CAD build for the part. Positions are in the model's coordinates, mm. A direction names the side the tool comes from. Give positions to 0.01 mm unless a question says otherwise; leave off trailing zeros. Loops run counter-clockwise (first coordinate to the right, second up) from the corner with the lowest first, then second, coordinate; pieces in that order, holes last. Notation, with made-up numbers: M 77.25,29.5 L 112.25,29.5 A19 ccw 112.25,48.5 Z; hole C 81.25,14 d9. An arc over 180 degrees is marked long. Answer as CSV lines item,"result".
```python
from build123d import *

# Parameters (mm, degrees)
SKETCH3_R          = 3
CUT_EXTRUDE1_DEPTH = 5


with BuildPart() as part:
    # Sketch1 → Revolve1 (revolve)
    with BuildSketch(Plane.XY, mode=Mode.PRIVATE) as revolve1_sk:
        Polygon((-15.060768988, 23.176328976), (-19, 22.481736265), (-19, 19.651328976), (-10.35, -0.323671024), (-8.6, -0.323671024), (-8.6, -6.823671024), (-5.6, -6.823671024), (-5.6, 3.426328976), (-3, 3.426328976), (-3, -1.573671024), (0, -1.573671024), (0, 23.176328976), align=None)
    revolve(revolve1_sk.sketch.rotate(Axis((0, -1.573671024, 0), (0, 1, 0)), 270), axis=Axis((0, -1.573671024, 0), (0, 1, 0)))

    # Sketch3 → Cut-Extrude1 (cut)
    with BuildSketch(Plane.XZ.offset(1.573671024)):
        Circle(SKETCH3_R)
    extrude(amount=-CUT_EXTRUDE1_DEPTH, mode=Mode.SUBTRACT)


solid = part.part
```
Q1. Cut at A-A (z = 0). Write the cut outline in (x, y), and give its area (3 significant figures).
Solution:
outline,"M -19,19.65 L -10.35,-0.32 L -8.6,-0.32 L -8.6,-6.82 L -5.6,-6.82 L -5.6,3.43 L 5.6,3.43 L 5.6,-6.82 L 8.6,-6.82 L 8.6,-0.32 L 10.35,-0.32 L 19,19.65 L 19,22.48 L 15.06,23.18 L -15.06,23.18 L -19,22.48 Z"
area,"714 mm²"
Q2. Wall check: line 1 (X direction, y = -4, z = 0); line 2 (X direction, y = 1.5, z = 0); line 3 (Z direction, x = -4.5, y = 0.5). Give the ranges that are in metal, low to high. Write a range as [from, to].
Solution:
line 1,"x = [-8.6, -5.6], [5.6, 8.6]"
line 2,"x = [-11.14, -5.6], [5.6, 11.14]"
line 3,"z = [-9.72, -3.33], [3.33, 9.72]"
Q3. Cut at C-C (y = -1). Write the cut outline in (x, z), and give its area (3 significant figures).
Solution:
outline,"C 0,0 d17.2; hole C 0,0 d11.2"
area,"134 mm²"
Q4. Cut at B-B (x = 0). Write the cut outline in (y, z), and give its area (3 significant figures).
Solution:
outline,"M -6.82,-8.6 L -0.32,-8.6 L -0.32,-10.35 L 19.65,-19 L 22.48,-19 L 23.18,-15.06 L 23.18,15.06 L 22.48,19 L 19.65,19 L -0.32,10.35 L -0.32,8.6 L -6.82,8.6 L -6.82,5.6 L 3.43,5.6 L 3.43,-5.6 L -6.82,-5.6 Z"
area,"714 mm²"
Q5. Mould opens along Z. For faces 1 (the cylindrical face through (5.233, -3.619, 6.825)), 2 (the cylindrical face through (-0.246, -1.627, 5.595)), 3 (the flat face through (6, -6.824, 0)) say: released by +Z, released by -Z, zero draft, split by the parting line, or undercut.
Solution:
face 1,"split by the parting line"
face 2,"undercut"
face 3,"zero draft"
Q6. Cut at D-D (y = 12.25). Write the cut outline in (x, z), and give its area (3 significant figures).
Solution:
outline,"C 0,0 d31.59"
area,"784 mm²"
Q7. Pin check, flat tips, straight feed: P1, Ø4, axis at y = 16, z = -11.5, coming from the -X side; P2, Ø8, axis at y = 5, z = 9.5, coming from the +X side; P3, Ø12, axis at x = 13.5, y = -1, coming from the -Z side. Stop position of each tip, or through.
Solution:
P1,"stops at x = -14.96"
P2,"stops at x = 12.18"
P3,"stops at z = -7.75"
Q8. Which spindle directions (+Z, -Z, +X, -X, +Y, -Y) get a long thin tool onto all of the face, cutting with end or side? Do faces 4 (the cylindrical face through (11.56, 21.05, 15.08)), 5 (the flat face through (0, 3.426, 0)). Say none if no direction does.
Solution:
face 4,"+Y, -Y"
face 5,"-Y"
